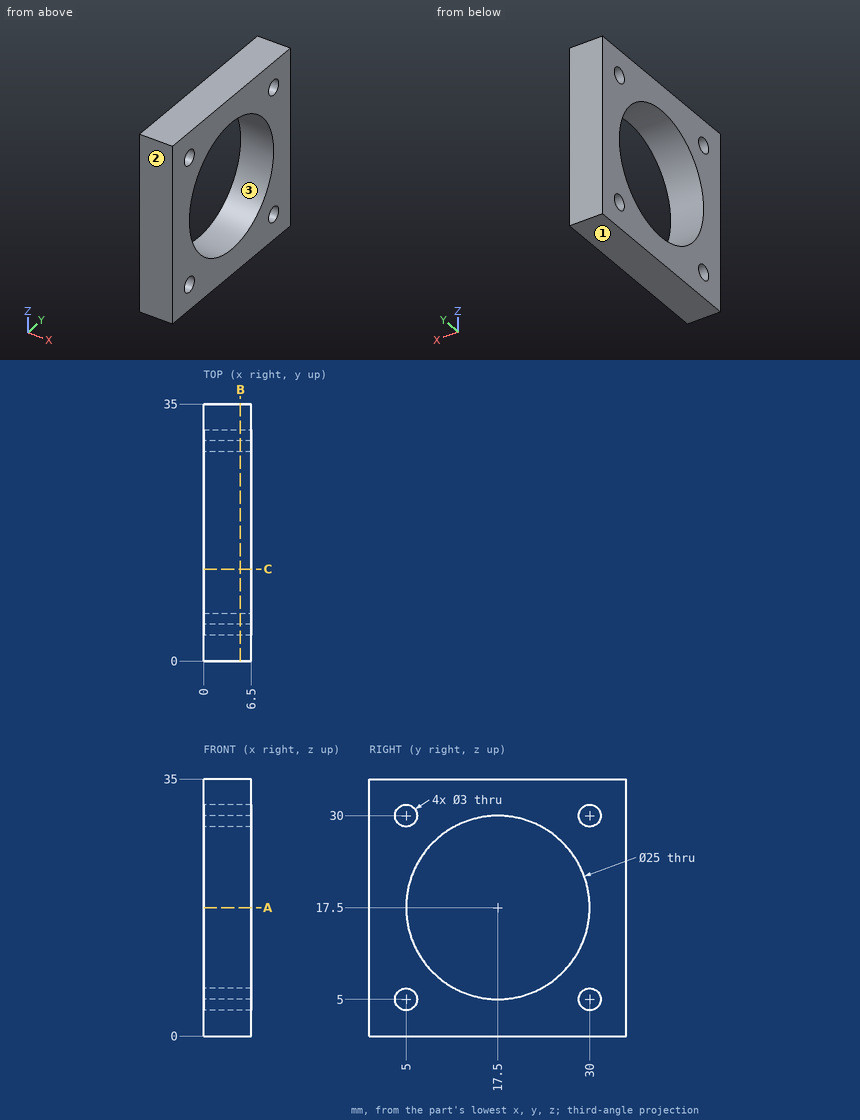
Study the drawing (mm; zero at the part's minimum x, y, z) and answer. Round coordinates to 2 decimals unless told otherwise and drop trailing zeros. Loops run counter-clockwise (first coordinate to the right, second up) from the corner with the lowest first, then second, coordinate; pieces in that order, holes last. Notation, with made-up numbers: (15, -34) -> (27, -34) arc R31 cw to (27, 0) -> close; hole circle Ø2 at (53.25, 17). An arc over 180 degrees is marked (long way). Write each question's results on one line, items separated by ' | '. Start each with the question number.
1. Section B-B (x = 5) is taken. Determine the outline of the cut face in (y, z).
2. Given pin 1 Ø2.5 at (y, z) = (5, 30) entering from +X; pin 2 Ø5 at (y, z) = (30, 5) entering from -X, each flat-ended and moving along its own axis, determine where each tip first touches the part or whether it passes through.
3. Section C-C (y = 12.5) is taken. Determine the outline of the cut face in (x, z), plus the area to 3 significant figures.
4. For a pull along Y with two mould halves and no side action, classify the marked faces 1, 2 and 3 as +Y half, -Y half, draft (parallel to the pull), parting line (faces both ways), or undercut.
5. Find the intervals of material crossed by probe 1 along Z at (x, y) = (3.75, 17.5); probe 2 along Y at (x, z) = (4.5, 4), in increasing order. Write a range as from..to.
6. Section A-A (z = 17.5) is taken. Determine the outline of the cut face in (x, y).
Evaluation:
1) outline: (0, 0) -> (35, 0) -> (35, 35) -> (0, 35) -> close; hole circle Ø3 at (5, 5); hole circle Ø3 at (5, 30); hole circle Ø25 at (17.5, 17.5); hole circle Ø3 at (30, 5); hole circle Ø3 at (30, 30)
2) pin 1: passes through | pin 2: stops at x = 0
3) outline: (0, 0) -> (6.5, 0) -> (6.5, 6.04) -> (0, 6.04) -> close; (0, 28.96) -> (6.5, 28.96) -> (6.5, 35) -> (0, 35) -> close | area: 78.6 mm2
4) face 1: draft | face 2: -Y half | face 3: undercut
5) probe 1: z = 0..5, 30..35 | probe 2: y = 0..3.88, 6.12..28.88, 31.12..35
6) outline: (0, 0) -> (6.5, 0) -> (6.5, 5) -> (0, 5) -> close; (0, 30) -> (6.5, 30) -> (6.5, 35) -> (0, 35) -> close
